Here's the drawing with two shaded views (mm, measured from the low corner). I have some questions. Coordinates: 2 decimals unless noted, no trailing zeros. Loops run counter-clockwise (first coordinate to the right, second up) from the corner with the lowest first, then second, coordinate; pieces in that order, holes last. Notation, with made-up numbers: (32, 19.5) - (83, 19.5) arc R27 ccw to (83, 42.5) - close; hole circle Ø5 at (-17, -34.75). An arc over 180 degrees is marked (long way). Use a Markdown table: item, result.
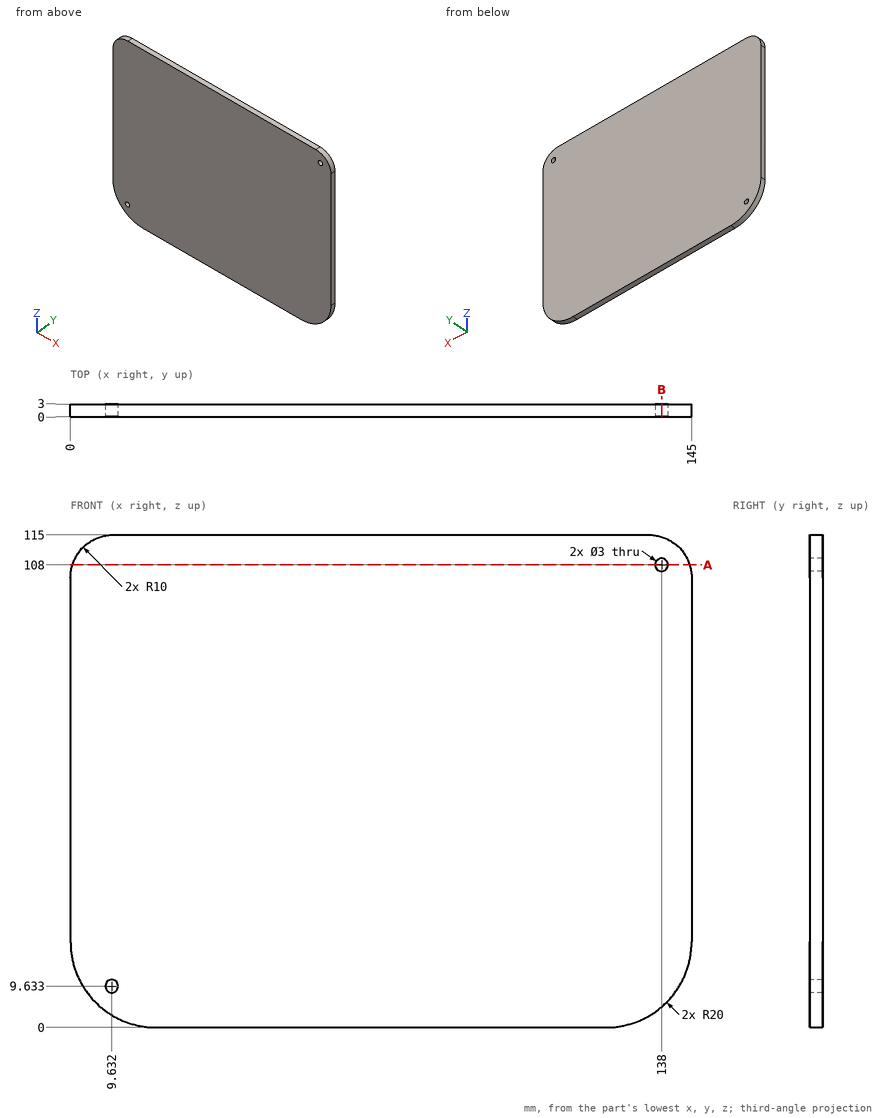
Q1. Please list where these lines run through material, in increasing order: L1, parallel to Z at x = 138, y = 2.35; L2, parallel to Z at x = 10, y = 2.2; L3, parallel to X at y = 1.1, z = 109 (1 decimal). Write a range as from..to.
Check values:
| item | result |
|---|---|
| L1 | 4.8..106.5, 109.5..114.54 |
| L2 | 2.68..8.18, 11.09..115 |
| L3 | 0.8..136.9, 139.1..144.2 |
Q2. I want a section at B-B, the plane x = 138. Write out the boundary of the cut face in (y, z), then the cut area to 3 significant figures.
Check values:
| item | result |
|---|---|
| outline | (0, 4.8) - (3, 4.8) - (3, 106.5) - (0, 106.5) - close; (0, 109.5) - (3, 109.5) - (3, 114.54) - (0, 114.54) - close |
| area | 320 mm^2 |
Q3. I want a section at A-A, the plane z = 108. Write out the boundary of the cut face in (x, y), then the cut area to 3 significant figures.
Check values:
| item | result |
|---|---|
| outline | (0.46, 0) - (136.5, 0) - (136.5, 3) - (0.46, 3) - close; (139.5, 0) - (144.54, 0) - (144.54, 3) - (139.5, 3) - close |
| area | 423 mm^2 |
